Read the model definition and answer for the solid it produces. Units are mm, in the model's axes. Face numbers are marked on the shaded views. Round coordinates to 2 decimals unless told otherwise and drop trailing zeros. Order: outer loops, then holes, each group sorted by start corner. A loop starts at its lowest first (then second) coordinate and runs counter-clockwise, first axis right, second up. Notation, with made-up numbers: (-35.75, 89) - (-12.75, 89) arc R22 cw to (-12.75, 118) - close; hole circle Ø5 at (31.5, 21.5). An arc over 180 degrees is marked (long way). One line per question, with ' | ' between items. Start each with the question number.
1) Straight lines are drawn through the part: line 1 (Y direction, x = 7, z = 4); line 2 (Y direction, x = 8, z = 3.25); line 3 (X direction, y = 7, z = 6.5). For each, find the intervals that lie inside material, in ascending order. Write a range as from..to.
2) Flat-ended cylindrical pins translate along their axes: pin 1 (1.5 mm diameter, centred on y = -1.5, z = 8.5, fed in from +X); pin 2 (1 mm diameter, centred on x = 13.5, z = 3.5, fed in from +Y). Find the tip coordinate at first contact, or state that the pin passes through.
3) The part is cut by section B-B, the plane x = 2.5. Give the vertices of the cut face in (y, z).
4) The mould has two halves that part along X. Classify the marked faces 1, 2 and 3: pulls with the +X half, pulls with the -X half, needs draft (parallel to the pull), parting line crosses it, or undercut.
5) The part is cut by section A-A, the plane z = 4.5. Count the separate pieces of the cut face and the enclosed holes in it, plus the area to 3 significant figures.
from build123d import *

# Parameters (mm, degrees)
SKETCH_1_R          = 11.5
EXTRUDE_1_DEPTH     = 10
SKETCH_2_R          = 1.6
CUT_EXTRUDE_1_DEPTH = 10


with BuildPart() as part:
    # 草圖1 → 填料-伸長1 (new body)
    with BuildSketch(Plane.XY):
        with BuildLine():
            ThreePointArc((0, 55), (-2.5, 57.5), (-5, 55))
            Line((-5, 55), (-10, 27.5))
            Line((-10, 27.5), (-10, -5))
            Line((-10, -5), (-4.5, -13))
            ThreePointArc((-4.5, -13), (-1.131727984, -4.868272016), (7, -1.5))
            Line((7, -1.5), (0, 0))
            add(Edge.make_bspline(
                [(0, 55), (-10, 27.5), (0, 0)],
                knots=[0, 0, 0, 1, 1, 1], degree=2))
        make_face()
        with Locations((7, -13)):
            Circle(SKETCH_1_R)
        with BuildLine():
            Line((8.124176937, 0.490227063), (7, -1.5))
            ThreePointArc((7, -1.5), (8.798996348, -1.641584083), (10.553695435, -2.062850063))
            Line((10.553695435, -2.062850063), (10.099553619, 0.177358133))
            Line((10.099553619, 0.177358133), (8.124176937, 0.490227063))
        make_face()
        with BuildLine():
            Line((14.154758721, -1.508288742), (12.24642256, -2.766474199))
            ThreePointArc((12.24642256, -2.766474199), (13.782706526, -3.713187189), (15.151977747, -4.888572333))
            Line((15.151977747, -4.888572333), (15.769856601, -2.687889877))
            Line((15.769856601, -2.687889877), (14.154758721, -1.508288742))
        make_face()
        with BuildLine():
            Line((18.609459232, -6.037927296), (16.337287066, -6.286947769))
            ThreePointArc((16.337287066, -6.286947769), (17.272482302, -7.830270089), (17.954734932, -9.500888316))
            Line((17.954734932, -9.500888316), (19.508542695, -7.824445957))
            Line((19.508542695, -7.824445957), (18.609459232, -6.037927296))
        make_face()
        with BuildLine():
            Line((20.507102251, -12.101006797), (18.371554502, -11.286013939))
            ThreePointArc((18.371554502, -11.286013939), (18.467843668, -12.140603924), (18.5, -13))
            ThreePointArc((18.5, -13), (18.461094648, -13.945150505), (18.34464183, -14.883905981))
            Line((18.34464183, -14.883905981), (20.492142426, -14.100950847))
            Line((20.492142426, -14.100950847), (20.507102251, -12.101006797))
        make_face()
        with BuildLine():
            ThreePointArc((17.901164481, -16.662596478), (17.193996736, -18.322821671), (16.23581896, -19.85198133))
            Line((16.23581896, -19.85198133), (18.504011675, -20.134964287))
            Line((18.504011675, -20.134964287), (19.429719792, -18.362095289))
            Line((19.429719792, -18.362095289), (17.901164481, -16.662596478))
        make_face()
        with BuildLine():
            ThreePointArc((15.029723408, -21.232468766), (13.643022341, -22.387238901), (12.092748017, -23.310864059))
            Line((12.092748017, -23.310864059), (13.98204893, -24.597456304))
            Line((13.98204893, -24.597456304), (15.614612218, -23.442148071))
            Line((15.614612218, -23.442148071), (15.029723408, -21.232468766))
        make_face()
        with BuildLine():
            ThreePointArc((10.389684506, -23.989087267), (8.628879877, -24.384056849), (6.827966819, -24.498713171))
            Line((6.827966819, -24.498713171), (7.922245347, -26.505534551))
            Line((7.922245347, -26.505534551), (9.902081321, -26.222251095))
            Line((9.902081321, -26.222251095), (10.389684506, -23.989087267))
        make_face()
        with BuildLine():
            ThreePointArc((5.003045957, -24.32528916), (3.255966224, -23.873463619), (1.601077028, -23.153897318))
            Line((1.601077028, -23.153897318), (1.659311339, -25.438932616))
            Line((1.659311339, -25.438932616), (3.55034849, -26.090068925))
            Line((3.55034849, -26.090068925), (5.003045957, -24.32528916))
        make_face()
    extrude(amount=EXTRUDE_1_DEPTH)

    # 草圖2 → 除料-伸長1 (cut)
    with BuildSketch(Plane.XY.offset(10)):
        with Locations((7, -5)):
            Circle(SKETCH_2_R)
        with Locations((7, -21)):
            Circle(SKETCH_2_R)
        with Locations((7, -13)):
            Circle(SKETCH_2_R)
    extrude(amount=-CUT_EXTRUDE_1_DEPTH, mode=Mode.SUBTRACT)


solid = part.part
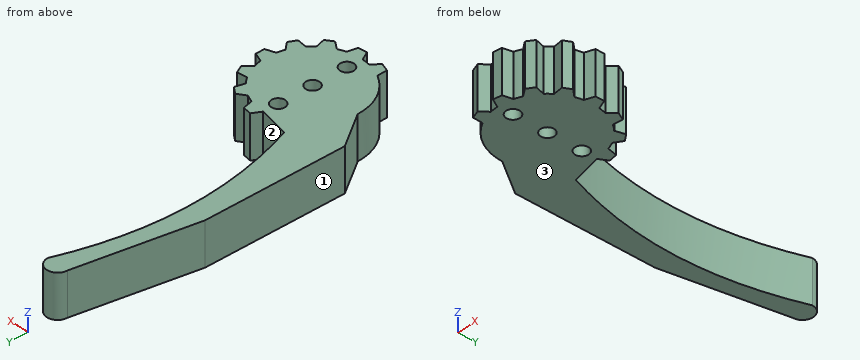
Values:
1) line 1: y = -24.81..-22.6, -19.4..-14.6, -11.4..-6.6, -3.4..-1.5 | line 2: y = -26.49..-22.25, -19.75..-14.25, -11.75..-6.25, -3.75..0.27 | line 3: x = -10..-2.22
2) pin 1: stops at x = 15.17 | pin 2: stops at y = -1.61
3) outline: (-25.73, 0) - (-0.54, 0) - (-0.54, 10) - (-25.73, 10) - close
4) face 1: pulls with the -X half | face 2: undercut | face 3: needs draft
5) separate pieces: 1 | enclosed holes: 3 | area: 834 mm^2
